Source: CAD feature listing. Evaluate the final solid. Frame: model axes, mm. Face numbers are marked on the shaded views. A direction names the side the tool comes from. Coordinates: 2 decimals unless noted, no trailing zeros. Write each loop counter-clockwise with the first axis right and the second up, starting at its lowest first coordinate (ties: lowest second). Pieces come first, ordered by that corner, then holes. Notation, with made-up numbers: (74, 20.5) - (90, 20.5) arc R29 ccw to (90, 51.5) - close; hole circle Ø3 at (73, 16.5). An arc over 180 degrees is marked (long way). One line per item, written item: value.
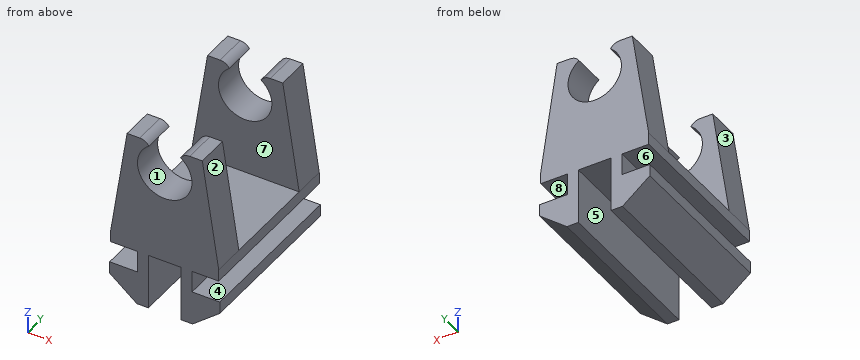
from build123d import *

# Parameters (mm, degrees)
F1_DEPTH     = 15
F3_DEPTH     = 25
F7_W         = 9.9
F7_H         = 3
F8_DEPTH     = 10
F10_DEPTH    = 3
F12_DEPTH    = 3
F13_T1_DEPTH = 7.2559990627
F13_T3_DEPTH = 7.2193706768


# Not quite as in the source:
# - a fillet or chamfer that OpenCascade refuses, or shapes differently, is made with other operations: its cross-section is extruded or revolved along the edge and cut away or added
# - a feature of the source that left no trace in its solid (it failed there, or was rolled back) is left out


with BuildPart() as f1:
    # F0 (on Front) → F1 (new body)
    with BuildSketch(Plane.XZ):
        Polygon((-2.5, 0.55), (-5.05, 0.55), (-5.05, -0.55), (-2.55, -2.55), (-1.5, -2.55), (-1.5, 2.55), (0, 2.55), (1.5, 2.55), (1.5, -2.55), (2.55, -2.55), (5.05, -0.55), (5.05, 0.55), (2.5, 0.55), (2.5, 2.55), (4.95, 2.55), (4.95, 3.65), (-4.95, 3.65), (-4.95, 2.55), (-2.5, 2.55), align=None)
    extrude(amount=F1_DEPTH)

    # F7 (on face) → F8 (join)
    with BuildSketch(Plane.XY.offset(3.65)):
        with Locations((0, -13.5)):
            Rectangle(F7_W, F7_H)
        with Locations((0, -1.5)):
            Rectangle(F7_W, F7_H)
    extrude(amount=F8_DEPTH)

    # F9 (on face) → F10 (cut, through all)
    with BuildSketch(Plane.XZ.offset(3)):
        with BuildLine():
            Line((-1.45, 13.65), (-1.45, 13.1748417658))
            ThreePointArc((-1.45, 13.1748417658), (0, 8.75), (1.45, 13.1748417658))
            Line((1.45, 13.1748417658), (1.45, 13.65))
            Line((1.45, 13.65), (-1.45, 13.65))
        make_face()
        Polygon((-4.95, 3.65), (-3.45, 13.65), (-4.95, 13.65), align=None)
        Polygon((4.95, 13.65), (3.45, 13.65), (4.95, 3.65), align=None)
    extrude(amount=-F10_DEPTH, mode=Mode.SUBTRACT)

    # F11 (on face) → F12 (cut, through all)
    with BuildSketch(Plane(origin=(0, -12, 0), x_dir=(-1, 0, 0), z_dir=(0, 1, 0))):
        with BuildLine():
            Line((-1.45, 13.65), (-1.45, 13.1865411854))
            ThreePointArc((-1.45, 13.1865411854), (0, 8.65), (1.45, 13.1865411854))
            Line((1.45, 13.1865411854), (1.45, 13.65))
            Line((1.45, 13.65), (-1.45, 13.65))
        make_face()
        Polygon((4.95, 13.65), (3.45, 13.65), (4.95, 3.65), align=None)
        Polygon((-4.95, 3.65), (-3.45, 13.65), (-4.95, 13.65), align=None)
    extrude(amount=-F12_DEPTH, mode=Mode.SUBTRACT)

    # F13: fillet of radius 1 on 4 edges, made by hand

    # F13_s2 → F13_t1 (cut)
    with BuildSketch(Plane.XZ.offset(-2.1279995313)):
        with BuildLine():
            ThreePointArc((1.45, 13.1748417658), (1.8137789296, 13.5231671563), (2.3011998125, 13.65))
            Line((2.3011998125, 13.65), (1.45, 13.65))
            Line((1.45, 13.65), (1.45, 13.1748417658))
        make_face()
        with BuildLine():
            ThreePointArc((-2.3011998125, 13.65), (-1.8137789296, 13.5231671563), (-1.45, 13.1748417658))
            Line((-1.45, 13.1748417658), (-1.45, 13.65))
            Line((-1.45, 13.65), (-2.3011998125, 13.65))
        make_face()
    extrude(amount=F13_T1_DEPTH, mode=Mode.SUBTRACT)

    # F13_s4 → F13_t3 (cut)
    with BuildSketch(Plane.XZ.offset(9.8903146616)):
        with BuildLine():
            ThreePointArc((1.45, 13.1865411854), (1.8124913279, 13.5265104636), (2.2938741354, 13.65))
            Line((2.2938741354, 13.65), (1.45, 13.65))
            Line((1.45, 13.65), (1.45, 13.1865411854))
        make_face()
        with BuildLine():
            ThreePointArc((-2.2938741354, 13.65), (-1.8124913279, 13.5265104636), (-1.45, 13.1865411854))
            Line((-1.45, 13.1865411854), (-1.45, 13.65))
            Line((-1.45, 13.65), (-2.2938741354, 13.65))
        make_face()
    extrude(amount=F13_T3_DEPTH, mode=Mode.SUBTRACT)


with BuildPart() as f3:
    # F2 (on face) → F3 (new body)
    with BuildSketch(Plane.XZ.offset(15)):
        with BuildLine():
            Line((-4.95, 3.65), (-4.0832418439, 3.65))
            Line((-4.0832418439, 3.65), (-0.75, 6.847274811))
            Line((-0.75, 6.847274811), (-0.75, 3.65))
            Line((-0.75, 3.65), (0.75, 3.65))
            Line((0.75, 3.65), (0.75, 6.828679691))
            Line((0.75, 6.828679691), (3.917720968, 3.65))
            Line((3.917720968, 3.65), (4.7647876878, 3.65))
            Line((4.7647876878, 3.65), (0.75, 7.6786768362))
            Line((0.75, 7.6786768362), (0.75, 7.9286768362))
            ThreePointArc((0.75, 7.9286768362), (0.6035533906, 8.2822302268), (0.25, 8.4286768362))
            Line((0.25, 8.4286768362), (-0.25, 8.4286768362))
            ThreePointArc((-0.25, 8.4286768362), (-0.6035533906, 8.2822302268), (-0.75, 7.9286768362))
            Line((-0.75, 7.9286768362), (-0.75, 7.6786768362))
            Line((-0.75, 7.6786768362), (-4.95, 3.65))
        make_face()
    extrude(amount=-F3_DEPTH)


solid = f1.part
1) Contact query for flat-ended pins moving along their axis: P1, Ø1, axis at y = -8.5, z = 1.5, coming from the -X side; P2, Ø1.3, axis at x = 3, y = -9, coming from the +Z side; P3, Ø0.9, axis at y = -7.5, z = 3, coming from the +X side. Output: stop coordinate, or through.
Values found:
P1: x = -2.5
P2: z = 3.65
P3: x = 4.95
2) Draft query along X for the marked faces 1, 2, 3 and 4. Return one class per face: released by +X, released by -X, zero draft, split by the parting line, or undercut.
Values found:
face 1: undercut
face 2: released by +X
face 3: released by -X
face 4: zero draft
3) Section query B-B on y = -7.25. Output: boundary loops of the cut face in (x, z).
Values found:
outline: (-5.05, -0.55) - (-2.55, -2.55) - (-1.5, -2.55) - (-1.5, 2.55) - (1.5, 2.55) - (1.5, -2.55) - (2.55, -2.55) - (5.05, -0.55) - (5.05, 0.55) - (2.5, 0.55) - (2.5, 2.55) - (4.95, 2.55) - (4.95, 3.65) - (-4.95, 3.65) - (-4.95, 2.55) - (-2.5, 2.55) - (-2.5, 0.55) - (-5.05, 0.55) - close
4) Section query C-C on z = 9.5. Output: boundary loops of the cut face in (x, y), then the cut area to 3 significant figures.
Values found:
outline: (-4.07, -15) - (-1.88, -15) - (-1.88, -12) - (-4.07, -12) - close; (-4.07, -3) - (-1.76, -3) - (-1.76, 0) - (-4.07, 0) - close; (1.76, -3) - (4.07, -3) - (4.07, 0) - (1.76, 0) - close; (1.88, -15) - (4.07, -15) - (4.07, -12) - (1.88, -12) - close
area: 27.0 mm2
5) Section query D-D on x = -1.75. Output: boundary loops of the cut face in (y, z), then the cut area to 3 significant figures.
Values found:
outline: (-15, -2.55) - (0, -2.55) - (0, 9.49) - (-3, 9.49) - (-3, 3.65) - (-12, 3.65) - (-12, 9.36) - (-15, 9.36) - close; (-15, 12.94) - (-12, 12.94) - (-12, 13.49) - (-15, 13.49) - close; (-3, 12.91) - (0, 12.91) - (0, 13.48) - (-3, 13.48) - close
area: 131 mm2
6) Material intervals for line 1 (Y direction, x = -3.75, z = 9.75); line 2 (X direction, y = -5.75, z = -0.5); line 3 (X direction, y = -11, z = 2.25), sorted ascending.
Values found:
line 1: -15 to -12, -3 to 0
line 2: -5.05 to -1.5, 1.5 to 5.05
line 3: -2.5 to -1.5, 1.5 to 2.5
7) Section query A-A on x = 0. Output: boundary loops of the cut face in (y, z), then the cut area to 3 significant figures.
Values found:
outline: (-15, 2.55) - (0, 2.55) - (0, 8.75) - (-3, 8.75) - (-3, 3.65) - (-12, 3.65) - (-12, 8.65) - (-15, 8.65) - close
area: 46.8 mm2
8) Reachability of the marked faces 5, 6, 7 and 8 from +Z, -Z, +X, -X, +Y, -Y: full face, straight path, thin tool, end or side. Return the list, or none.
Values found:
face 5: -Z, +Y, -Y
face 6: -X, +Y, -Y
face 7: +Z, +X, -X
face 8: +X, +Y, -Y
